Source: three-view drawing plus pictorial views. Frame: mm from the lowest corner of the part. Round coordinates to 2 decimals unless told otherwise and drop trailing zeros. Order: outer loops, then holes, each group sorted by start corner. A loop starts at its lowest first (then second) coordinate and runs counter-clockwise, first axis right, second up. Notation, with made-up numbers: M -34.75,-8.75 L -14.75,-8.75 A21 cw -14.75,5.25 Z; hole C -31.75,60.25 d3. An arc over 180 degrees is marked long. Return JSON: item names as keys, results as strings. Group by question number.
Q1. Ray query, probe 1 along Z at (x, y) = (102.5, 63). Return the intervals inside material, ascending.
Q2. Cut plane B-B on x = 90. Output: boundary loops of the cut face in (y, z).
Q3. Contact query for flat-ended pins moving along their axis: pin 1 (2 mm diameter, centred on y = 48.5, z = 4, fed in from -X); pin 2 (0.9 mm diameter, centred on x = 36, y = 24.5, fed in from -Z); pin 3 (5 mm diameter, centred on y = 28.5, z = 3, fed in from +X); pin 4 (6 mm diameter, centred on y = 14, z = 4, fed in from -X). Output: stop coordinate, or through.
Q4. Cut plane A-A on z = 5. Count the separate pieces of the cut face and the enclosed holes in it, and give its area (3 significant figures).
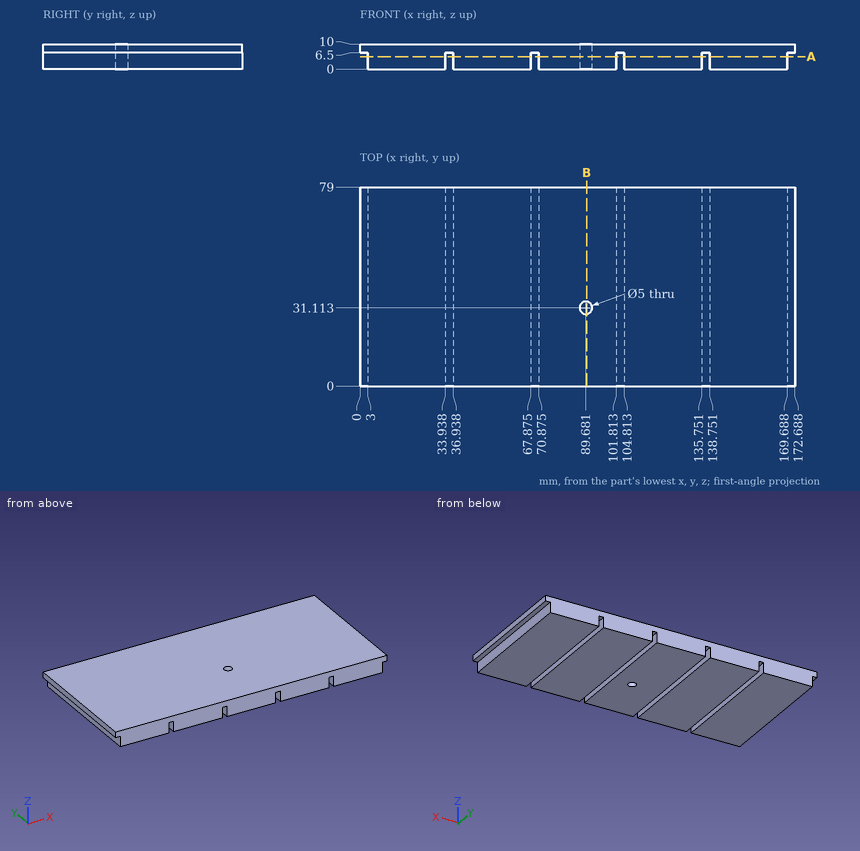
Result sheet:
{
 "1": {"probe 1": "z = 6.5 to 10"},
 "2": {"outline": "M 0,0 L 28.63,0 L 28.63,10 L 0,10 Z; M 33.59,0 L 79,0 L 79,10 L 33.59,10 Z"},
 "3": {"pin 1": "stops at x = 3", "pin 2": "stops at z = 6.5", "pin 3": "stops at x = 169.69", "pin 4": "stops at x = 0"},
 "4": {"separate pieces": "5", "enclosed holes": "1", "area": "12,200 mm²"}
}
